Could you check a few things on this model? Use its own coordinates, in mm. Face numbers are marked on the shaded views. A direction names the side the tool comes from. Coordinates: 2 decimals unless noted, no trailing zeros. Loops run counter-clockwise (first coordinate to the right, second up) from the corner with the lowest first, then second, coordinate; pieces in that order, holes last. Notation, with made-up numbers: M 11,-11 L 51,-11 A20 ccw 51,8 Z; hole C 38.5,29.5 d2. An arc over 180 degrees is marked long. Use one line per item in the form item = value. Start each with the question number.
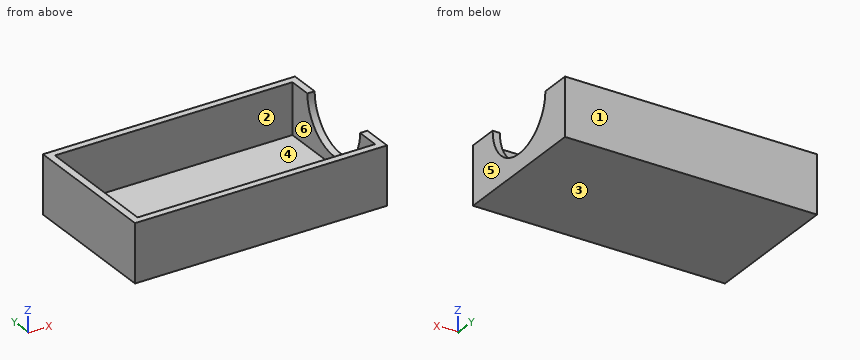
```python
from build123d import *

# Parameters (mm, degrees)
F0_W     = 88.392
F0_H     = 50.292
F1_DEPTH = 20.32
F2_T     = -2.54
F4_DEPTH = 25.4


with BuildPart() as f1:
    # F0 (on Top) → F1 (new body)
    with BuildSketch(Plane.XY):
        with Locations((44.196, 25.146)):
            Rectangle(F0_W, F0_H)
    extrude(amount=F1_DEPTH)

    # F2
    f2_openings = [f1.faces().sort_by_distance(p)[0] for p in [
        (44.196, 25.146, 20.32),
    ]]
    offset(amount=F2_T, openings=f2_openings)

    # F3 (on face) → F4 (cut)
    with BuildSketch(Plane.YZ.offset(88.392)):
        with BuildLine():
            ThreePointArc((10.742303, 20.32), (25.146, 5.916303), (39.549697, 20.32))
            Line((39.549697, 20.32), (10.742303, 20.32))
        make_face()
    extrude(amount=-F4_DEPTH, mode=Mode.SUBTRACT)


solid = f1.part
```
Item 1: I want a section at C-C (z = 13.75). Write out the boundary of the cut face in (x, y).
Item 2: Thinking about a two-plate mould opening in Y: for the marked faces 1, 2, 3 and 4, which applies, pulls with the +Y half, pulls with the -Y half, needs draft (parallel to the pull), parting line crosses it, or undercut?
Item 3: I want a section at D-D (z = 7.75). Write out the boundary of the cut face in (x, y), plus the area to 3 significant figures.
Item 4: Please list where these lines run through material, in increasing order: line 1 along X through (y, z) = (45, 10.5); line 2 along Y through (x, z) = (14.5, 16.25); line 3 along X through (y, z) = (24, 9.75).
Item 5: For the marked faces 5 and 6, which set-ups out of +Z, -Z, +X, -X, +Y, -Y let a thin tool reach every point of the face, with its end or its side?
Item 6: I want a section at B-B (y = 41). Write out the boundary of the cut face in (x, z).
Item 7: I'm going to push flat-ended pins straight in: P1, Ø9, axis at y = 18, z = 14.5, coming from the +X side; P2, Ø13.5, axis at x = 64, y = 25.5, coming from the +Z side. Where does each tip first touch, or does it pass through?
Item 8: I want a section at A-A (x = 40.5). Write out the boundary of the cut face in (y, z).
Worked answers:
q1.outline = M 0,0 L 88.39,0 L 88.39,12.33 L 85.85,12.33 L 85.85,2.54 L 2.54,2.54 L 2.54,47.75 L 85.85,47.75 L 85.85,37.96 L 88.39,37.96 L 88.39,50.29 L 0,50.29 Z
q2.face_1 = pulls with the +Y half
q2.face_2 = undercut
q2.face_3 = needs draft
q2.face_4 = undercut
q3.outline = M 0,0 L 88.39,0 L 88.39,18.11 L 85.85,18.11 L 85.85,2.54 L 2.54,2.54 L 2.54,47.75 L 85.85,47.75 L 85.85,32.18 L 88.39,32.18 L 88.39,50.29 L 0,50.29 Z
q3.area = 643 mm²
q4.line_1 = 0 to 2.54, 85.85 to 88.39
q4.line_2 = 0 to 2.54, 47.75 to 50.29
q4.line_3 = 0 to 2.54
q5.face_5 = +Z, -Z, +X, +Y, -Y
q5.face_6 = +Z
q6.outline = M 0,0 L 88.39,0 L 88.39,20.32 L 85.85,20.32 L 85.85,2.54 L 2.54,2.54 L 2.54,20.32 L 0,20.32 Z
q7.P1 = 2.54
q7.P2 = 2.54
q8.outline = M 0,0 L 50.29,0 L 50.29,20.32 L 47.75,20.32 L 47.75,2.54 L 2.54,2.54 L 2.54,20.32 L 0,20.32 Z
